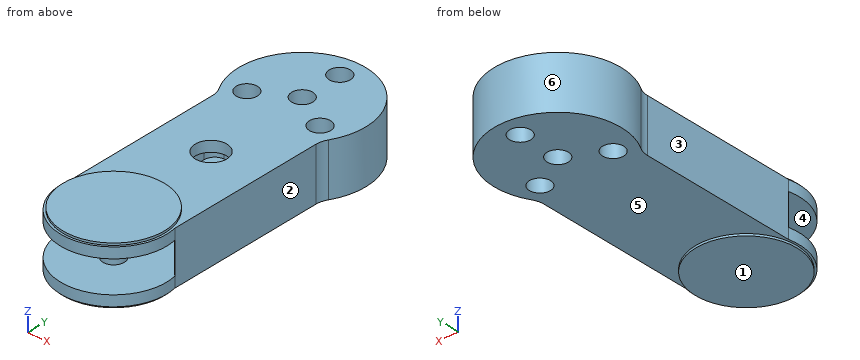
```python
from build123d import *

# Parameters (mm, degrees)
BOSS_EXTRU_1_DEPTH      = 25
ENL_V_MAT_EXTRU_6_DEPTH = 15
ESQUISSE7_R             = 10
ENL_V_MAT_EXTRU_7_DEPTH = 263.603726785
ESQUISSE8_R             = 48
BOSS_EXTRU_2_DEPTH      = 2
BOSS_EXTRU_3_START      = 2
ESQUISSE9_R             = 48
BOSS_EXTRU_3_DEPTH      = 2
ESQUISSE11_R            = 15
ENL_V_MAT_EXTRU_8_DEPTH = 20
ESQUISSE12_R            = 10
BOSS_EXTRU_4_DEPTH      = 30


with BuildPart() as part:
    # Esquisse1 → Boss.-Extru.1 (new, symmetric)
    with BuildSketch(Plane.XY):
        with BuildLine():
            Line((48.961575437, -40.549982901), (48.961575437, -190.58313224))
            ThreePointArc((48.961575437, -190.58313224), (0, -250.7203967), (-48.961575437, -190.58313224))
            Line((-48.961575437, -190.58313224), (-48.961575437, -40.549982901))
            ThreePointArc((-48.961575437, -40.549982901), (-49.663805136, -35.296787549), (-51.721181578, -30.412487176))
            ThreePointArc((-51.721181578, -30.412487176), (0, 60), (51.721181578, -30.412487176))
            ThreePointArc((51.721181578, -30.412487176), (49.663805136, -35.296787549), (48.961575437, -40.549982901))
        make_face()
    extrude(amount=BOSS_EXTRU_1_DEPTH, both=True)

    # Esquisse6 → Enlèv. mat.-Extru.6 (cut, symmetric)
    with BuildSketch(Plane.XY):
        with BuildLine():
            Line((-48.961575437, -190.58313224), (-44.819439813, -186.440996616))
            ThreePointArc((-44.819439813, -186.440996616), (-40.483984787, -179.95252964), (-38.961575437, -172.298860992))
            Line((-38.961575437, -172.298860992), (-38.961575437, -60.549982901))
            ThreePointArc((-38.961575437, -60.549982901), (-36.032643249, -53.478915089), (-28.961575437, -50.549982901))
            Line((-28.961575437, -50.549982901), (28.961575437, -50.549982901))
            ThreePointArc((28.961575437, -50.549982901), (36.032643249, -53.478915089), (38.961575437, -60.549982901))
            Line((38.961575437, -60.549982901), (38.961575437, -172.298860992))
            ThreePointArc((38.961575437, -172.298860992), (40.483984787, -179.95252964), (44.819439813, -186.440996616))
            Line((44.819439813, -186.440996616), (48.961575437, -190.58313224))
            Line((48.961575437, -190.58313224), (84.871492003, -248.547724845))
            Line((84.871492003, -248.547724845), (0, -290.851549547))
            Line((0, -290.851549547), (-95.233900293, -248.547724845))
            Line((-95.233900293, -248.547724845), (-48.961575437, -190.58313224))
        make_face()
    extrude(amount=ENL_V_MAT_EXTRU_6_DEPTH, both=True, mode=Mode.SUBTRACT)

    # Esquisse7 → Enlèv. mat.-Extru.7 (cut, through all)
    with BuildSketch(Plane.XY.offset(25)):
        Circle(ESQUISSE7_R)
        with Locations((0, 40)):
            Circle(ESQUISSE7_R)
        with Locations((34.641016151, -20)):
            Circle(ESQUISSE7_R)
        with Locations((-34.641016151, -20)):
            Circle(ESQUISSE7_R)
    extrude(amount=-ENL_V_MAT_EXTRU_7_DEPTH, mode=Mode.SUBTRACT)

    # Esquisse8 → Boss.-Extru.2 (add)
    with BuildSketch(Plane.XY.offset(25)):
        with Locations(Location((0, -200.7203967, 0), (0, 0, 180))):
            Circle(ESQUISSE8_R)
    extrude(amount=BOSS_EXTRU_2_DEPTH)

    # Esquisse9 → Boss.-Extru.3 (add)
    with BuildSketch(Plane(origin=(0, 0, -25), x_dir=(-1, 0, 0), z_dir=(0, 0, -1)).offset(BOSS_EXTRU_3_START)):
        with Locations((0, -200.7203967)):
            Circle(ESQUISSE9_R)
    extrude(amount=-BOSS_EXTRU_3_DEPTH)

    # Esquisse11 → Enlèv. mat.-Extru.8 (cut)
    with BuildSketch(Plane.XY.offset(25)):
        with Locations((0, -97.061157092)):
            Circle(ESQUISSE11_R)
    extrude(amount=-ENL_V_MAT_EXTRU_8_DEPTH, mode=Mode.SUBTRACT)

    # Esquisse12 → Boss.-Extru.4 (add)
    with BuildSketch(Plane.XY.offset(-15)):
        with Locations(Location((0, -200.7203967, 0), (0, 0, 180))):
            Circle(ESQUISSE12_R)
    extrude(amount=BOSS_EXTRU_4_DEPTH)


solid = part.part
```
Here's how the part is built. I have some questions about the finished solid (model axes, mm). Face numbers are marked on the shaded views. A direction names the side the tool comes from. Give positions to 0.01 mm unless a question says otherwise; leave off trailing zeros. Write each loop counter-clockwise with the first axis right and the second up, starting at its lowest first coordinate (ties: lowest second). Pieces come first, ordered by that corner, then holes.
(1) If I drill on L1, parallel to Y at x = 0, z = -2; L2, parallel to Y at x = 0, z = 23; L3, parallel to Z at x = 36, y = -87, over which ranges is the centre line in solid material (lowest first)?
Output values:
L1: y = -210.72 to -190.72, -50.55 to -10, 10 to 30, 50 to 60
L2: y = -250.72 to -112.06, -82.06 to -10, 10 to 30, 50 to 60
L3: z = -25 to -15, 15 to 25
(2) On a 3-axis mill with a long thin cutter (end or side, diameter ignored), from which of +Z, -Z, +X, -X, +Y, -Y can I reach the whole of each face in a straight line? I mean the marked faces 1, 2 and 3. Say none if no direction works.
Output values:
face 1: -Z, +X, -X, +Y, -Y
face 2: +Z, -Z, +X
face 3: +Z, -Z, -X
(3) Imagine slicing it at D-D, the plane x = -21. Write out the boundary of the cut face in (y, z).
Output values:
outline: (-246.1, -25) - (-243.88, -25) - (-243.88, -27) - (-157.56, -27) - (-157.56, -25) - (56.2, -25) - (56.2, 25) - (-157.56, 25) - (-157.56, 27) - (-243.88, 27) - (-243.88, 25) - (-246.1, 25) - (-246.1, 15) - (-50.55, 15) - (-50.55, -15) - (-246.1, -15) - close
(4) Imagine slicing it at A-A, the plane y = 0. Write out the boundary of the cut face in (x, z), and give its area (3 significant figures).
Output values:
outline: (-60, -25) - (-10, -25) - (-10, 25) - (-60, 25) - close; (10, -25) - (60, -25) - (60, 25) - (10, 25) - close
area: 5,000 mm2
(5) Will these pins go through, and if not, where does the flat tip stop? pin 1 (1 mm diameter, centred on y = -56, z = 6, fed in from -X); pin 2 (1 mm diameter, centred on y = 1.5, z = 18, fed in from +X); pin 3 (6 mm diameter, centred on y = 2.5, z = 12.5, fed in from -X); pin 4 (4 mm diameter, centred on x = 27.5, z = -17.5, fed in from -Y).
Output values:
pin 1: stops at x = -48.96
pin 2: stops at x = 59.99
pin 3: stops at x = -60
pin 4: stops at y = -243.73
(6) Imagine slicing it at B-B, the plane z = -1.5. Write out the boundary of the cut face in (x, y).
Output values:
outline: (-51.72, -30.41) arc R20 cw to (-48.96, -40.55) - (-48.96, -190.58) - (-44.82, -186.44) arc R20 ccw to (-38.96, -172.3) - (-38.96, -60.55) arc R10 cw to (-28.96, -50.55) - (28.96, -50.55) arc R10 cw to (38.96, -60.55) - (38.96, -172.3) arc R20 ccw to (44.82, -186.44) - (48.96, -190.58) - (48.96, -40.55) arc R20 cw to (51.72, -30.41) arc R60 ccw (long way) to start; circle Ø20 at (0, -200.72); hole circle Ø20 at (-34.64, -20); hole circle Ø20 at (0, 0); hole circle Ø20 at (0, 40); hole circle Ø20 at (34.64, -20)
(7) Thinking about a two-plate mould opening in Z: for the marked faces 4, 5 and 6, which applies, pulls with the +Z half, pulls with the -Z half, needs draft (parallel to the pull), parting line crosses it, or undercut?
Output values:
face 4: undercut
face 5: pulls with the -Z half
face 6: needs draft
(8) Imagine slicing it at C-C, the plane x = 0. Count the separate pieces of the cut face and the enclosed holes in it, and give its area (3 significant figures).
Output values:
separate pieces: 3
enclosed holes: 0
area: 8,210 mm2
